```python
from build123d import *

# Parameters (mm, degrees)
SKETCH1_W                = 22.5
SKETCH1_H                = 7
BOSS_EXTRUDE1_DEPTH      = 1.5
SKETCH2_R                = 1.475
BOSS_EXTRUDE2_DEPTH      = 11.5
SKETCH3_R                = 1.05
BOSS_EXTRUDE3_DEPTH      = 9
BOSS_EXTRUDE4_DEPTH      = 6
BOSS_EXTRUDE4_DEPTH_BACK = 1.5
SKETCH4_W                = 22.5
SKETCH4_H                = 2.5
SKETCH4_H_2              = 7
SKETCH8_W                = 22.5
SKETCH8_H                = 9.5
BOSS_EXTRUDE7_DEPTH      = 2.61
BOSS_EXTRUDE8_DEPTH      = 7.76
BOSS_EXTRUDE8_DEPTH_BACK = 1.5
SKETCH9_R                = 2.4
SKETCH11_W               = 9.5
SKETCH11_H               = 3
BOSS_EXTRUDE9_DEPTH      = 4.5
SKETCH16_W               = 1.5
SKETCH16_H               = 9.5
CUT_EXTRUDE2_DEPTH       = 1.5
SKETCH19_W               = 3
SKETCH19_H               = 5
BOSS_EXTRUDE10_DEPTH     = 10
SKETCH20_W               = 13
SKETCH20_H               = 2
CUT_EXTRUDE3_DEPTH       = 7.5
FILLET1_SIZE             = 4
FILLET1_SIZE_2           = 1.5
FILLET2_R                = 1.5
FILLET3_R                = 1.5
FILLET4_R                = 2
FILLET5_R                = 0.5
FILLET6_SIZE             = 5
FILLET6_SIZE_2           = 2.5
FILLET7_R                = 2.5
FILLET8_R                = 2.5
FILLET9_R                = 2.5
FILLET10_R               = 2.5


# Some blends are built 0.0001 mm under size
with BuildPart() as part:
    # Sketch1 → Boss-Extrude1 (new body)
    with BuildSketch(Plane(origin=(0, 0, 0), x_dir=(1, 0, 0), z_dir=(0, 1, 0))):
        with Locations((-28.93578967, -21.079480712)):
            Rectangle(SKETCH1_W, SKETCH1_H)
    extrude(amount=BOSS_EXTRUDE1_DEPTH)

    # Sketch2 → Boss-Extrude2 (add)
    with BuildSketch(Plane(origin=(0, 1.5, 0), x_dir=(1, 0, 0), z_dir=(0, 1, 0))):
        with Locations(Location((-37.53578967, -19.579480712, 0), (0, 0, 90))):
            Circle(SKETCH2_R)
        with Locations(Location((-20.33578967, -19.579480712, 0), (0, 0, 90))):
            Circle(SKETCH2_R)
    extrude(amount=BOSS_EXTRUDE2_DEPTH)

    # Sketch3 → Boss-Extrude3 (add)
    with BuildSketch(Plane(origin=(0, 1.5, 0), x_dir=(1, 0, 0), z_dir=(0, 1, 0))):
        with Locations(Location((-37.88578967, -23.029480712, 0), (0, 0, 90))):
            Circle(SKETCH3_R)
        with Locations(Location((-19.98578967, -23.029480712, 0), (0, 0, 90))):
            Circle(SKETCH3_R)
    extrude(amount=BOSS_EXTRUDE3_DEPTH)

    # Sketch4 → Boss-Extrude4 (add, two sides: drawn at the far end of the back side and taken through both)
    with BuildSketch(Plane(origin=(0, 0, 0), x_dir=(-1, 0, 0), z_dir=(0, -1, 0)).offset(-BOSS_EXTRUDE4_DEPTH_BACK)):
        with Locations((28.93578967, -25.829480712)):
            Rectangle(SKETCH4_W, SKETCH4_H)
        with Locations((28.93578967, -21.079480712)):
            Rectangle(SKETCH4_W, SKETCH4_H_2)
    extrude(amount=BOSS_EXTRUDE4_DEPTH + BOSS_EXTRUDE4_DEPTH_BACK)

    # Sketch8 → Boss-Extrude7 (add)
    with BuildSketch(Plane(origin=(0, 1.5, 0), x_dir=(1, 0, 0), z_dir=(0, 1, 0))):
        with Locations((-28.93578967, -22.329480712)):
            Rectangle(SKETCH8_W, SKETCH8_H)
    extrude(amount=BOSS_EXTRUDE7_DEPTH)

    # Sketch9 → Boss-Extrude8 (add, two sides: drawn at the far end of the back side and taken through both)
    with BuildSketch(Plane(origin=(0, -6, 0), x_dir=(-1, 0, 0), z_dir=(0, -1, 0)).offset(-BOSS_EXTRUDE8_DEPTH_BACK)):
        with Locations(Location((28.81078967, -25.489480712, 0), (0, 0, 90))):
            Circle(SKETCH9_R)
        with Locations(Location((28.81078967, -17.519480712, 0), (0, 0, 90))):
            Circle(SKETCH9_R)
    extrude(amount=BOSS_EXTRUDE8_DEPTH + BOSS_EXTRUDE8_DEPTH_BACK)

    # Sketch11 → Boss-Extrude9 (add)
    with BuildSketch(Plane(origin=(-17.68578967, 0, 0), x_dir=(0, 0, -1), z_dir=(1, 0, 0))):
        with Locations((-22.329480712, -2.09)):
            Rectangle(SKETCH11_W, SKETCH11_H)
    extrude(amount=BOSS_EXTRUDE9_DEPTH)

    # Sketch16 → Cut-Extrude2 (cut)
    with BuildSketch(Plane(origin=(0, -0.59, 0), x_dir=(1, 0, 0), z_dir=(0, 1, 0))):
        with Locations((-15.43578967, -22.329480712)):
            Rectangle(SKETCH16_W, SKETCH16_H)
    extrude(amount=-CUT_EXTRUDE2_DEPTH, mode=Mode.SUBTRACT)

    # Sketch19 → Boss-Extrude10 (add)
    with BuildSketch(Plane.XY.offset(27.079480712)):
        with Locations((-22.43578967, -3.5)):
            Rectangle(SKETCH19_W, SKETCH19_H)
        with Locations((-35.43578967, -3.5)):
            Rectangle(SKETCH19_W, SKETCH19_H)
    extrude(amount=BOSS_EXTRUDE10_DEPTH)

    # Sketch20 → Cut-Extrude3 (cut)
    with BuildSketch(Plane.XY.offset(37.079480712)):
        with Locations((-28.93578967, -3.5)):
            Rectangle(SKETCH20_W, SKETCH20_H)
    extrude(amount=-CUT_EXTRUDE3_DEPTH, mode=Mode.SUBTRACT)

    # Fillet1
    # an asymmetric fillet: 4, 1.5 mm, written as the material it adds along each edge
    with BuildSketch(Plane(origin=(-17.68578967, -0.59, 17.579480712), x_dir=(0, 1, 0), z_dir=(0, 0, 1))) as fillet1_piece_1:
        with BuildLine():
            Bezier((FILLET1_SIZE, 0), (0, 0), (0, -FILLET1_SIZE_2), weights=[1, 0.707106781, 1])
            Line((0, -FILLET1_SIZE_2), (0, 0))
            Line((0, 0), (FILLET1_SIZE, 0))
        make_face()
    extrude(amount=9.5)

    # Fillet2
    fillet2_edges = [part.edges().sort_by_distance(p)[0] for p in [
        (-17.68578967, -3.59, 22.329480712),
    ]]
    fillet(fillet2_edges, radius=FILLET2_R)

    # Fillet3
    fillet3_edges = [part.edges().sort_by_distance(p)[0] for p in [
        (-13.18578967, -3.59, 22.329480712),
    ]]
    fillet(fillet3_edges, radius=FILLET3_R)

    # Fillet4
    fillet4_edges = [part.edges().sort_by_distance(p)[0] for p in [
        (-28.81078967, -4.5, 17.579480712),
    ]]
    fillet(fillet4_edges, radius=FILLET4_R)

    # Fillet5
    fillet5_edges = [part.edges().sort_by_distance(p)[0] for p in [
        (-28.81078967, -4.5, 27.079480712),
    ]]
    fillet(fillet5_edges, radius=FILLET5_R)

    # Fillet6
    # an asymmetric fillet: 5, 2.5 mm, written as the material it takes off along each edge
    with BuildSketch(Plane(origin=(-40.18578967, 16.61, 17.579480712), x_dir=(1, 0, 0), z_dir=(0, -1, 0))) as fillet6_piece_1:
        with BuildLine():
            Bezier((FILLET6_SIZE, 0), (0, 0), (0, FILLET6_SIZE_2), weights=[1, 0.707106781, 1])
            Line((0, FILLET6_SIZE_2), (0, 0))
            Line((0, 0), (FILLET6_SIZE, 0))
        make_face()
    extrude(amount=35.11, mode=Mode.SUBTRACT)

    # Fillet7
    fillet7_edges = [part.edges().sort_by_distance(p)[0] for p in [
        (-36.93578967, -6, 32.079480712),
    ]]
    fillet(fillet7_edges, radius=FILLET7_R)

    # Fillet8
    fillet8_edges = [part.edges().sort_by_distance(p)[0] for p in [
        (-36.93578967, -1, 32.079480712),
    ]]
    fillet(fillet8_edges, radius=FILLET8_R - 0.0001)  # a hair under: the kernel refuses the full size

    # Fillet9
    fillet9_edges = [part.edges().sort_by_distance(p)[0] for p in [
        (-20.93578967, -1, 32.079480712),
    ]]
    fillet(fillet9_edges, radius=FILLET9_R)

    # Fillet10
    fillet10_edges = [part.edges().sort_by_distance(p)[0] for p in [
        (-20.93578967, -6, 32.079480712),
    ]]
    fillet(fillet10_edges, radius=FILLET10_R - 0.0001)  # a hair under: the kernel refuses the full size


solid = part.part
```
Geometry check sheet. Reference: the model listing, model coordinates, mm. A direction names the side the tool comes from. Give positions to 0.01 mm unless a question says otherwise; leave off trailing zeros. Loops run counter-clockwise (first coordinate to the right, second up) from the corner with the lowest first, then second, coordinate; pieces in that order, holes last. Notation, with made-up numbers: M -36.75,42 L -7.75,42 A13 ccw -7.75,56 Z; hole C 7.5,65.5 d4. An arc over 180 degrees is marked long. Write item = value, one per line.
(1) Sectioned sample at D-D, the plane y = 8. Record the cut outline in (x, z) (3 decimals).
Answer below:
outline = C -37.536,19.579 d2.95; C -37.886,23.029 d2.1; C -20.336,19.579 d2.95; C -19.986,23.029 d2.1
(2) Sectioned sample at C-C, the plane y = -7.75. Record the cut outline in (x, z).
Answer below:
outline = C -28.81,17.52 d4.8; C -28.81,25.49 d4.8
(3) Gauge pin test, flat ends, axial feed: pin 1 Ø1 at (x, y) = (-25, 3.5) entering from -Z; pin 2 Ø1 at (y, z) = (8.5, 22.5) entering from +X; pin 3 Ø1.2 at (x, z) = (-34.5, 35) entering from -Y; pin 4 Ø5 at (y, z) = (-0.5, 29) entering from +X. Record the tip position at first contact, or that the pin passes through.
Answer below:
pin_1 = 17.58
pin_2 = -18.94
pin_3 = -6
pin_4 = -13.19
(4) Tool access check on faces 4 (the face through (-14.686, -1, 22)), 5 (the face through (-23, -3, 29.579)), 6 (the face through (-21.6, -5.2, 32.1)), 7 (the face through (-38.927, 7.26, 23.166)). Record the directions out of +Z, -Z, +X, -X, +Y, -Y that give a thin tool (end or side, any length) a straight path to the whole face; none if there is none.
Answer below:
face_4 = +Z, -Z, +Y
face_5 = +Z
face_6 = +Z, +X, -Y
face_7 = +Y
(5) Release check for a two-part mould opening along X. For faces 1 (the face through (-13.186, -1, 22)), 2 (the face through (-38, 10.5, 23)), 3 (the face through (-15, -2.09, 22)) record: released by +X, released by -X, zero draft, split by the parting line, or undercut.
Answer below:
face_1 = released by +X
face_2 = zero draft
face_3 = undercut
(6) Material ranges on line 1 (Y direction, x = -23.5, z = 32); line 2 (Z direction, x = -25.25, y = 2.75); line 3 (Z direction, x = -28.5, y = -11.5), recorded low to high. Write a range as [from, to].
Answer below:
line_1 = [-6, -4.5], [-2.5, -1]
line_2 = [17.58, 27.08]
line_3 = [15.14, 19.9], [23.11, 27.87]
(7) Sectioned sample at B-B, the plane x = -29.5. Record the cut outline in (y, z).
Answer below:
outline = M -13.76,15.22 L -4.5,15.22 L -4.5,15.58 A2 cw -2.5,17.58 L 4.11,17.58 L 4.11,27.08 L -4,27.08 A0.5 cw -4.5,27.58 L -4.5,27.79 L -13.76,27.79 L -13.76,23.19 L -6,23.19 L -6,19.82 L -13.76,19.82 Z
